from build123d import *

# Parameters (mm, degrees)
SKETCH_2_W      = 191.4
SKETCH_2_H      = 231.6
EXTRUDE_1_DEPTH = 2
SKETCH_3_W      = 185
SKETCH_3_H      = 2
EXTRUDE_2_DEPTH = 2.5
SKETCH_4_W      = 191.4
SKETCH_4_H      = 2
EXTRUDE_3_DEPTH = 37.4
SKETCH_7_R      = 5
EXTRUDE_5_DEPTH = 10


with BuildPart() as part:
    # 草图2 → 凸台-拉伸1 (new body)
    with BuildSketch(Plane(origin=(0, 0, 0), x_dir=(1, 0, 0), z_dir=(0, 1, 0))):
        Rectangle(SKETCH_2_W, SKETCH_2_H)
    extrude(amount=EXTRUDE_1_DEPTH)

    # 草图3 → 凸台-拉伸2 (add)
    with BuildSketch(Plane(origin=(0, 2, 0), x_dir=(1, 0, 0), z_dir=(0, 1, 0))):
        with Locations((0, 114.8)):
            Rectangle(SKETCH_3_W, SKETCH_3_H)
        with Locations((0, -114.8)):
            Rectangle(SKETCH_3_W, SKETCH_3_H)
    extrude(amount=EXTRUDE_2_DEPTH)

    # 草图4 → 凸台-拉伸3 (add)
    with BuildSketch(Plane(origin=(0, 4.5, 0), x_dir=(1, 0, 0), z_dir=(0, 1, 0))):
        with Locations((0, 114.8)):
            Rectangle(SKETCH_4_W, SKETCH_4_H)
        with Locations((0, -114.8)):
            Rectangle(SKETCH_4_W, SKETCH_4_H)
    extrude(amount=EXTRUDE_3_DEPTH)

    # 草图7 → 凸台-拉伸5 (add)
    with BuildSketch(Plane.XY.offset(115.8)):
        with Locations(Location((0, 20.95, 0), (0, 0, 180))):
            Circle(SKETCH_7_R)
    extrude(amount=EXTRUDE_5_DEPTH)


solid = part.part
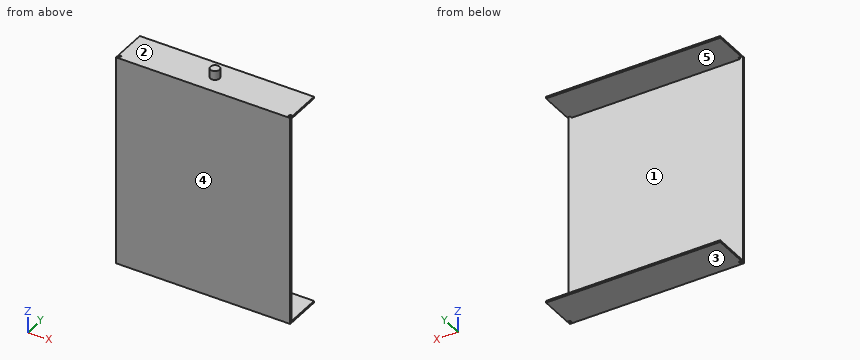
Input: part model. Units: mm. Frame: model coordinates. Face numbers are marked on the shaded views. A direction names the side the tool comes from. Coordinates: 2 decimals unless noted, no trailing zeros. Order: outer loops, then holes, each group sorted by start corner. A loop starts at its lowest first (then second) coordinate and runs counter-clockwise, first axis right, second up. Notation, with made-up numbers: M -28.5,64 L 23.5,64 A25 ccw 23.5,94 Z; hole C -13.5,16 d2. An arc over 180 degrees is marked long. One line per question, with ' | ' between items.
Item 1: Reachability of the marked faces 4 and 5 from +Z, -Z, +X, -X, +Y, -Y: full face, straight path, thin tool, end or side. Return the list, or none.
Geometry results:
face 4: +Z, -Z, +X, -X, -Y | face 5: +X, -X, +Y
Item 2: Section D-D (z = -90.5). Output: boundary loops of the cut face in (x, y), then the cut area to 3 significant figures.
Geometry results:
outline: M -95.7,0 L 95.7,0 L 95.7,2 L -95.7,2 Z | area: 383 mm^2
Item 3: Section B-B (x = -44). Output: boundary loops of the cut face in (y, z), then the cut area to 3 significant figures.
Geometry results:
outline: M 0,-115.8 L 41.9,-115.8 L 41.9,-113.8 L 2,-113.8 L 2,113.8 L 41.9,113.8 L 41.9,115.8 L 0,115.8 Z | area: 623 mm^2
Item 4: Pin query (flat end, axial travel): pin 1 (21 mm diameter, centred on x = -18.5, y = 22, fed in from +Z); pin 2 (0.6 mm diameter, centred on x = -93.5, z = 115, fed in from -Y); pin 3 (1 mm diameter, centred on x = 46.5, z = -80.5, fed in from +Y); pin 4 (0.6 mm diameter, centred on y = 3, z = 114.5, fed in from -X). Return the tip coordinate at first contact, or that it passes through.
Geometry results:
pin 1: stops at z = 115.8 | pin 2: stops at y = 0 | pin 3: stops at y = 2 | pin 4: stops at x = -92.5
Item 5: Ray query, line 1 along Z through (x, y) = (-48, 18.5); line 2 along Y through (x, z) = (88.5, 67.5). Return the intervals inside material, ascending.
Geometry results:
line 1: z = -115.8 to -113.8, 113.8 to 115.8 | line 2: y = 0 to 2
Item 6: Section A-A (y = 20.95). Output: boundary loops of the cut face in (x, z).
Geometry results:
outline: M -95.7,-115.8 L 95.7,-115.8 L 95.7,-113.8 L -95.7,-113.8 Z; M -95.7,113.8 L 95.7,113.8 L 95.7,115.8 L 5,115.8 L 5,125.8 L -5,125.8 L -5,115.8 L -95.7,115.8 Z
Item 7: Section C-C (y = 7.5). Output: boundary loops of the cut face in (x, z).
Geometry results:
outline: M -95.7,-115.8 L 95.7,-115.8 L 95.7,-113.8 L -95.7,-113.8 Z; M -95.7,113.8 L 95.7,113.8 L 95.7,115.8 L -95.7,115.8 Z
Item 8: Draft query along Z for the marked faces 1, 2 and 3. Return one class per face: released by +Z, released by -Z, zero draft, split by the parting line, or undercut.
Geometry results:
face 1: undercut | face 2: released by +Z | face 3: released by -Z
